Geometry check sheet. Reference: the model listing, model coordinates, mm. A direction names the side the tool comes from. Round coordinates to 2 decimals unless told otherwise and drop trailing zeros. Loops run counter-clockwise (first coordinate to the right, second up) from the corner with the lowest first, then second, coordinate; pieces in that order, holes last.
```python
from build123d import *

# Parameters (mm, degrees)
CROQUIS1_R              = 6
CROQUIS1_R_2            = 3.5
SALIENTE_EXTRUIR1_DEPTH = 28
CROQUIS2_R              = 6
SALIENTE_EXTRUIR2_DEPTH = 5
CROQUIS3_R              = 2.75
SALIENTE_EXTRUIR3_DEPTH = 20
REDONDEO1_R             = 0.5
REDONDEO2_R             = 0.8
REDONDEO3_R             = 0.5


with BuildPart() as part:
    # Croquis1 → Saliente-Extruir1 (new body)
    with BuildSketch(Plane.XY):
        Circle(CROQUIS1_R)
        Circle(CROQUIS1_R_2, mode=Mode.SUBTRACT)
    extrude(amount=SALIENTE_EXTRUIR1_DEPTH)

    # Croquis2 → Saliente-Extruir2 (add)
    with BuildSketch(Plane.XY.offset(28)):
        Circle(CROQUIS2_R)
    extrude(amount=SALIENTE_EXTRUIR2_DEPTH)

    # Croquis3 → Saliente-Extruir3 (add)
    with BuildSketch(Plane.XY.offset(33)):
        Circle(CROQUIS3_R)
    extrude(amount=SALIENTE_EXTRUIR3_DEPTH)

    # Redondeo1
    redondeo1_edges = [part.edges().sort_by_distance(p)[0] for p in [
        (-6, 0, 33),
    ]]
    fillet(redondeo1_edges, radius=REDONDEO1_R)

    # Redondeo2
    redondeo2_edges = [part.edges().sort_by_distance(p)[0] for p in [
        (-6, 0, 0),
    ]]
    fillet(redondeo2_edges, radius=REDONDEO2_R)

    # Redondeo3
    redondeo3_edges = [part.edges().sort_by_distance(p)[0] for p in [
        (-2.75, 0, 53),
    ]]
    fillet(redondeo3_edges, radius=REDONDEO3_R)


solid = part.part
```
1) Sectioned sample at C-C, the plane z = 4. Record the cut outline in (x, y), then the cut area to 3 significant figures.
Report:
outline: circle Ø12 at (0, 0); hole circle Ø7 at (0, 0)
area: 74.6 mm2
2) Gauge pin test, flat ends, axial feed: pin 1 (2 mm diameter, centred on x = 4.5, z = 22, fed in from -Y); pin 2 (3 mm diameter, centred on x = 3, z = 17, fed in from +Y); pin 3 (5 mm diameter, centred on y = 4.5, z = 22, fed in from -X); pin 4 (1 mm diameter, centred on y = 4.5, z = 43.5, fed in from +X). Record the tip position at first contact, or that the pin passes through.
Report:
pin 1: stops at y = -4.87
pin 2: stops at y = 5.81
pin 3: stops at x = -5.66
pin 4: passes through
3) Sectioned sample at D-D, the plane z = 46. Record the cut outline in (x, y), then the cut area to 3 significant figures.
Report:
outline: circle Ø5.5 at (0, 0)
area: 23.8 mm2
4) Mould release check, pull along Y, two halves, no side actions. Record for faces 1 (the face through (0, 4, 0)), 2 (the face through (-0.596, -2.685, 42.614)), 3 (the face through (3.233, -1.341, 13.804)): +Y half, -Y half, draft (parallel to the pull), parting line (faces both ways), or undercut.
Report:
face 1: draft
face 2: parting line
face 3: undercut
5) Sectioned sample at A-A, the plane x = 0. Record the cut outline in (y, z), then the cut area to 3 significant figures.
Report:
outline: (-6, 0.8) arc R0.8 ccw to (-5.2, 0) - (-3.5, 0) - (-3.5, 28) - (3.5, 28) - (3.5, 0) - (5.2, 0) arc R0.8 ccw to (6, 0.8) - (6, 32.5) arc R0.5 ccw to (5.5, 33) - (2.75, 33) - (2.75, 52.5) arc R0.5 ccw to (2.25, 53) - (-2.25, 53) arc R0.5 ccw to (-2.75, 52.5) - (-2.75, 33) - (-5.5, 33) arc R0.5 ccw to (-6, 32.5) - close
area: 310 mm2
6) Access from +Z, -Z, +X, -X, +Y, -Y to the whole of each face (thin tool, end or side, straight path). Record for faces 4 (the face through (0, 0, 28)), 5 (the face through (-3, -1, 33)), 6 (the face through (0, 0, 53)).
Report:
face 4: -Z
face 5: +Z
face 6: +Z, +X, -X, +Y, -Y
7) Scan lines: line 1 along Y through (x, z) = (0, 10.5); line 2 along Z through (x, y) = (0.75, -4); line 3 along Z through (x, y) = (0.75, 1). Record each from-to range of solid material in increasing order.
Report:
line 1: y = -6 to -3.5, 3.5 to 6
line 2: z = 0 to 33
line 3: z = 28 to 53
